CAD build for the part. Positions are in the model's coordinates, mm. A direction names the side the tool comes from. Coordinates: 2 decimals unless noted, no trailing zeros. Loops run counter-clockwise (first coordinate to the right, second up) from the corner with the lowest first, then second, coordinate; pieces in that order, holes last. Notation, with made-up numbers: (70.5, 2.25) - (81.5, 2.25) arc R11 ccw to (81.5, 6.25) - close; hole circle Ø7 at (-2, 71.5). An arc over 180 degrees is marked (long way). Put each result on its own line as item: value.
```python
from build123d import *

# Parameters (mm, degrees)
F0_R     = 7.9375
F2_DEPTH = 2.54
F3_START = 2.54
F1_R     = 3.2004
F3_DEPTH = 2.4765
F4_R     = 0.508
F5_SIZE  = 0.508


with BuildPart() as f2:
    # F0 (on Top) → F2 (new body)
    with BuildSketch(Plane.XY):
        Circle(F0_R)
    extrude(amount=F2_DEPTH)

    # F1 (on Top) → F3 (join)
    with BuildSketch(Plane.XY.offset(F3_START)):
        Circle(F1_R)
    extrude(amount=F3_DEPTH)

    # F4
    f4_edges = [f2.edges().sort_by_distance(p)[0] for p in [
        (-3.2004, 0, 5.0165),
        (-7.9375, 0, 2.54),
    ]]
    fillet(f4_edges, radius=F4_R)

    # F5
    f5_edges = [f2.edges().sort_by_distance(p)[0] for p in [
        (-7.9375, 0, 0),
    ]]
    chamfer(f5_edges, length=F5_SIZE)


solid = f2.part
```
Q1. Slice it at A-A, the plane y = 0. Give the cut face in (x, z), then the cut area to 3 significant figures.
Determined:
outline: (-7.94, 0.51) - (-7.43, 0) - (7.43, 0) - (7.94, 0.51) - (7.94, 2.03) arc R0.51 ccw to (7.43, 2.54) - (3.2, 2.54) - (3.2, 4.51) arc R0.51 ccw to (2.69, 5.02) - (-2.69, 5.02) arc R0.51 ccw to (-3.2, 4.51) - (-3.2, 2.54) - (-7.43, 2.54) arc R0.51 ccw to (-7.94, 2.03) - close
area: 55.7 mm2
Q2. Tool access for faces 1 (the cylindrical face through (-2.54, -1.95, 3.51)), 2 (the flat face through (0, 0, 0)): list every direction of +Z, -Z, +X, -X, +Y, -Y with a clear straight run to the whole face (end or side of a thin tool).
Determined:
face 1: +Z
face 2: -Z, +X, -X, +Y, -Y
Q3. Wall check: L1, parallel to Z at x = -3, y = 2.5; L2, parallel to Y at x = -0.5, z = 2.3; L3, parallel to Y at x = -0.75, z = 2.45. Give the ranges that are in metal, low to high. Write a range as from..to.
Determined:
L1: 0..2.54
L2: -7.85..7.85
L3: -7.68..7.68
Q4. Slice it at C-C, the plane z = 2.8. Give the cut face in (x, y), then the cut area to 3 significant figures.
Determined:
outline: circle Ø6.4 at (0, 0)
area: 32.2 mm2
Q5. Pin check, flat tip, straight feed: pin 1 Ø5 at (x, y) = (-1, -6) entering from +Z. Stop position of the tip, or through.
Determined:
pin 1: z = 2.54
